For this review, take the finished solid that the model builds, in its own axes (mm). A direction names the side the tool comes from. Round coordinates to 2 decimals unless told otherwise and drop trailing zeros. Order: outer loops, then holes, each group sorted by start corner. A loop starts at its lowest first (then second) coordinate and runs counter-clockwise, first axis right, second up. Notation, with made-up numbers: (82, 72.25) - (91, 72.25) arc R13 ccw to (91, 80.25) - close; hole circle Ø9 at (38, -20.5). An arc over 180 degrees is marked (long way). Write each question's results on one line, items separated by ' | '. Start each with the question number.
(1) Insertion check: pin 1 Ø4 at (x, z) = (-0.5, -5) entering from +Y; pin 2 Ø0.6 at (x, z) = (-1, 5) entering from +Y; pin 3 Ø8 at (x, z) = (-8.5, -12) entering from -Y; pin 4 Ø5 at (x, y) = (0.5, 17) entering from +Z. Each pin has a flat end and moves straight along its axis. Give the tip position at first contact, or say it passes through.
(2) Take a section at C-C, the plane z = -9.25. Give the boundary of the cut face in (x, y).
(3) For L1, parallel to Y at x = -1, z = -5.25; L2, parallel to Y at x = 0.5, z = -11.25; L3, parallel to Z at x = -4.75, y = 16, list the stretches that pass through material, from the lowest coordinate up. Write a range as from..to.
(4) Take a section at B-B, the plane z = -2.5. Give the boundary of the cut face in (x, y), plus the area to 3 significant figures.
(5) Take a section at D-D, the plane z = 4. Give the boundary of the cut face in (x, y), plus the area to 3 significant figures.
(6) Take a section at A-A, the plane z = -5. Give the boundary of the cut face in (x, y), plus the area to 3 significant figures.
(7) Draft analysis for pull direction Z (two halves, no side actions). For faces 1 (the flat face through (-13.733, 12, -3)), 2 (the flat face through (2, 21, -0.554)), 3 (the cylindrical face through (-13.59, 12.318, -13.663)), 4 (the flat face through (2, 21, -6.554)), state which applies: pulls with the +Z half, pulls with the -Z half, needs draft (parallel to the pull), parting line crosses it, or undercut.
(8) For faces 5 (the flat face through (0.267, 21, -4)), 6 (the cylindrical face through (3.12, 12.32, -13.67)), list the 3-axis set-ups (+Z, -Z, +X, -X, +Y, -Y) from which the entire face can be reached by the end or side of a thin tool; tool diameter is ignored.
Autodesk Inventor part; units mm, degrees
ref_plane "YZ Plane" through (0, 0, 0) normal (1, 0, 0) x (0, 1, 0)
ref_plane "XZ Plane" through (0, 0, 0) normal (0, 1, 0) x (-1, 0, 0)
ref_plane "XY Plane" through (0, 0, 0) normal (0, 0, 1) x (1, 0, 0)
sketch "Sketch1" plane through (0, 0, 0) normal (0, 1, 0) x (-1, 0, 0)
  line L0 (5.232996, 7.4455) -> (-11.767004, 7.4455)
  line L1 (-11.767004, 7.4455) -> (-11.767004, -14.5545)
  line L2 (-11.767004, -14.5545) -> (5.232996, -14.5545)
  circle A0 centre (-3.267004, -3.5545) radius 3.5
  line L3 (5.232996, 7.4455) -> (5.232996, -14.5545)
  point P0 (0, 0)
  dimension "d2" = 22
  dimension "d3" = 17
  dimension "d8" = 7
  dimension "d10" = 11
  dimension "d11" = 8.5
extrude "Extrusion1" add sketch "Sketch1" along normal blind 20
sketch "Sketch2" plane through (0, 20, 0) normal (0, 1, 0) x (1, 0, 0)
  line L0 (-5.232996, -7.4455) -> (11.767004, -7.4455)
  line L1 (11.767004, -7.4455) -> (11.767004, 14.5545)
  line L2 (-5.232996, -7.4455) -> (11.767004, -7.4455)
  line L3 (11.767004, -7.4455) -> (11.767004, -4.9455)
  line L4 (11.767004, -4.9455) -> (-5.232996, -4.9455)
  line L5 (-5.232996, -4.9455) -> (-5.232996, -7.4455)
  line L6 (-5.232996, 14.5545) -> (-5.232996, -7.4455)
  line L7 (-5.232996, 14.5545) -> (11.767004, 14.5545)
  line L8 (11.767004, 14.5545) -> (11.767004, 12.0545)
  line L9 (11.767004, 12.0545) -> (-5.232996, 12.0545)
  line L10 (-5.232996, 12.0545) -> (-5.232996, 14.5545)
  line L11 (11.767004, 0.5545) -> (8.767004, 0.5545)
  line L12 (8.767004, 0.5545) -> (8.767004, 6.5545)
  line L13 (8.767004, 6.5545) -> (11.767004, 6.5545)
  line L14 (11.767004, 6.5545) -> (11.767004, 0.5545)
  line L15 (11.767004, 0.5545) -> (8.767004, 0.5545)
  line L16 (8.767004, 0.5545) -> (8.767004, 6.5545)
  line L17 (8.767004, 6.5545) -> (11.767004, 6.5545)
  line L18 (11.767004, 6.5545) -> (11.767004, 0.5545)
  point P0 (0, 0)
  dimension "d14" = 2.5
  dimension "d15" = 2.5
  dimension "d16" = 3
  dimension "d17" = 6
  dimension "d18" = 8
extrude "Extrusion2" add sketch "Sketch2" along normal blind 1 contours L5 L4 L1 L0 | L6 L7 L1 L9
sketch "Sketch3" plane through (0, 20, 0) normal (0, 1, 0) x (1, 0, 0)
  line L0 (11.767004, -4.9455) -> (11.767004, 12.0545)
  line L1 (11.767004, 0.5545) -> (8.767004, 0.5545)
  line L2 (8.767004, 0.5545) -> (8.767004, 6.5545)
  line L3 (8.767004, 6.5545) -> (11.767004, 6.5545)
  line L4 (11.767004, 6.5545) -> (11.767004, 0.5545)
  line L5 (-5.232996, -7.4455) -> (11.767004, -7.4455)
  point P0 (0, 0)
  dimension "d21" = 6
  dimension "d22" = 3
  dimension "d23" = 8
extrude "Extrusion3" add sketch "Sketch3" along normal blind 3
sketch "Sketch5" plane through (-5.232996, 0, -14.5545) normal (-1, 0, 0) x (0, 0, 1)
  line L0 (-21.5, -5) -> (43.5, -5)
  line L1 (11, -5) -> (11, 5)
  line L2 (0, 0) -> (0, 21)
  arc A0 (43.5, -5) -> (22, 3.943867) centre (11, -52.8125) ccw
  line L3 (2.5, 20) -> (19.5, 20)
  arc A1 (11, 5) -> (-21.5, -5) centre (11, -52.8125) ccw
  arc A2 (0, 3.943867) -> (-21.5, -5) centre (11, -52.8125) ccw
  line L4 (0, 0) -> (22, 0)
  line L5 (22, 0) -> (22, 3.943867)
  line L6 (22, 0) -> (0, 0)
  line L7 (0, 0) -> (0, 3.943867)
  arc A3 (22, 3.943867) -> (11, 5) centre (11, -52.8125) ccw
  line L8 (-15.777391, -378) -> (53.366362, -378)
  point P0 (14.5545, 0)
  dimension "d27" = 65
  dimension "d28" = 10
  dimension "d29" = 32.5
  dimension "d30" = 21.5
  dimension "d31" = 15
  dimension "d32" = 373
move or copy body "Move Body1" bodies to move or copy 1 copy no translate (-8.5, 0, 0)
revolve "Revolution1" cut sketch "Sketch5" angle 360 about axis through (-5.232996, -378, -30.331891) along (0, 0, 1)
fillet "Fillet2" radius 0.5 1 edges at (-5.233, 20, -12.0545)
fillet "Fillet3" radius 0.5 1 edges at (-5.233, 20, 4.9455)
sketch "Sketch6" plane through (3.267004, 21, -12.0545) normal (1, 0, 0) x (0, 0, -1)
  line L0 (-17, 0) -> (-19.5, 0)
  line L1 (-17, 0) -> (-18, 0)
  line L2 (-19.5, -17.150727) -> (-19.5, 0)
  line L3 (-18, 0) -> (-19.5, -17.150727)
  line L4 (-19.5, -17.150727) -> (-19.5, 0)
  line L5 (-19.5, 0) -> (-18, 0)
  line L6 (0, 0) -> (2.5, 0)
  line L7 (0, 0) -> (1, 0)
  line L8 (2.5, -17.150727) -> (2.5, 0)
  line L9 (1, 0) -> (2.5, -17.150727)
  line L10 (2.5, -17.150727) -> (2.5, 0)
  line L11 (2.5, 0) -> (1, 0)
  point P0 (-12.0545, -21)
  dimension "d40" = 1
  dimension "d41" = 1
extrude "Extrusion4" cut sketch "Sketch6" against normal up to next
fillet "Fillet4" radius 0.5 6 edges at (-5.233, 21, 5.9455) (3.267, 12.4246, 6.6955) (-13.733, 12.4246, 6.6955) (3.267, 12.4246, -13.8045) (-5.233, 21, -13.0545) (-13.733, 12.4246, -13.8045)
properties part number "upper_fender_spacer"
Results below:
1) pin 1: stops at y = 23 | pin 2: stops at y = 21 | pin 3: stops at y = 3.89 | pin 4: stops at z = 6.51
2) outline: (-13.73, 4.62) arc R382.72 cw to (3.27, 4.62) - (3.27, 20) - (-13.73, 20) - close
3) L1: y = 4.95..20 | L2: y = 4.44..20 | L3: z = -13.49..-7.02, -0.09..6.38
4) outline: (-13.73, 4.9) arc R382.99 cw to (-8.57, 4.98) - (-8.57, 20) - (-13.73, 20) - close; (-1.9, 4.98) arc R382.99 cw to (3.27, 4.9) - (3.27, 23) - (0.27, 23) - (0.27, 20) - (-1.9, 20) - close | area: 164 mm^2
5) outline: (-13.73, 4.41) arc R382.5 cw to (3.27, 4.41) - (3.27, 20) - (-13.73, 20) - close | area: 264 mm^2
6) outline: (-13.73, 4.89) arc R382.98 cw to (-8.42, 4.97) - (-8.42, 20) - (-13.73, 20) - close; (-2.05, 4.97) arc R382.98 cw to (3.27, 4.89) - (3.27, 23) - (0.27, 23) - (0.27, 20) - (-2.05, 20) - close | area: 169 mm^2
7) face 1: needs draft | face 2: undercut | face 3: pulls with the -Z half | face 4: undercut
8) face 5: -X, +Y | face 6: -Z, +X, +Y
